Can you work these out from the model? Positions are in its coordinate system, mm. Face numbers are marked on the shaded views. Give positions to 0.01 mm unless a question says otherwise; leave off trailing zeros. Loops run counter-clockwise (first coordinate to the right, second up) from the corner with the lowest first, then second, coordinate; pieces in that order, holes last. Notation, with made-up numbers: (0.25, -14) - (51.25, -14) arc R28 cw to (51.25, 22) - close; hole circle Ø4 at (83, 28). An arc over 180 degrees is marked (long way). Write item = value, one per line.
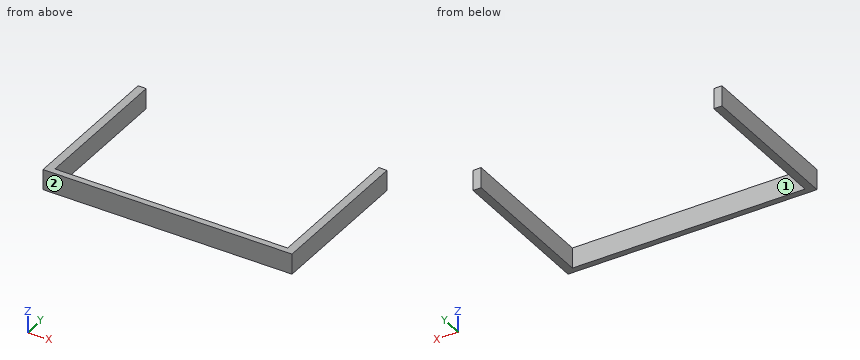
from build123d import *

# Parameters (mm, degrees)
SKETCH1_W             = 4
SKETCH1_H             = 75
BOSS_EXTRUDE1_DEPTH   = 10
BOSS_EXTRUDE1_2_DEPTH = 10
SKETCH3_W             = 122
SKETCH3_H             = 3
BOSS_EXTRUDE2_DEPTH   = 10


with BuildPart() as part:
    # Sketch1 → Boss-Extrude1 (new body)
    with BuildSketch(Plane.XY):
        with Locations((-59, 37.5)):
            Rectangle(SKETCH1_W, SKETCH1_H)
    extrude(amount=BOSS_EXTRUDE1_DEPTH)



with BuildPart() as body_2:
    # Sketch1 → Boss-Extrude1 2 (new body)
    with BuildSketch(Plane.XY):
        with Locations((59, 37.5)):
            Rectangle(SKETCH1_W, SKETCH1_H)
    extrude(amount=BOSS_EXTRUDE1_2_DEPTH)


with BuildPart() as part_1:
    add(part.part)

    add(body_2.part)  # Boss-Extrude2 merges body 2
    # Sketch3 → Boss-Extrude2 (add)
    with BuildSketch(Plane.XY):
        with Locations((0, 1.5)):
            Rectangle(SKETCH3_W, SKETCH3_H)
    extrude(amount=BOSS_EXTRUDE2_DEPTH)


solid = part_1.part
Q1. Imagine slicing it at A-A, the plane y = 17.5. Write out the boundary of the cut face in (x, z), then the cut area to 3 significant figures.
Output:
outline = (-61, 0) - (-57, 0) - (-57, 10) - (-61, 10) - close; (57, 0) - (61, 0) - (61, 10) - (57, 10) - close
area = 80.0 mm2
Q2. We'd pull the mould along X, two halves only. Please class the marked faces 1 and 2: released by +X, released by -X, zero draft, split by the parting line, or undercut.
Output:
face_1 = undercut
face_2 = zero draft
Q3. Imagine slicing it at B-B, the plane z = 8.75. Write out the boundary of the cut face in (x, y).
Output:
outline = (-61, 0) - (61, 0) - (61, 75) - (57, 75) - (57, 3) - (-57, 3) - (-57, 75) - (-61, 75) - close
Q4. For pin 1 (8 mm diameter, centred on x = -7, y = 9.5, fed in from -Z); pin 2 (6 mm diameter, centred on x = -21.5, z = 9, fed in from +Y), each with a flat end and sliding along its axis, tell me the tip position at first contact or that it passes through.
Output:
pin_1 = through
pin_2 = 3
Q5. I need wall thicknesses on L1, parallel to X at y = 54, z = 1; L2, parallel to Y at x = -5, z = 7. Which ranges of each line are inside material? Lowest first, please.
Output:
L1 = -61 to -57, 57 to 61
L2 = 0 to 3
Q6. Imagine slicing it at C-C, the plane x = 46.5. Write out the boundary of the cut face in (y, z), then the cut area to 3 significant figures.
Output:
outline = (0, 0) - (3, 0) - (3, 10) - (0, 10) - close
area = 30.0 mm2
